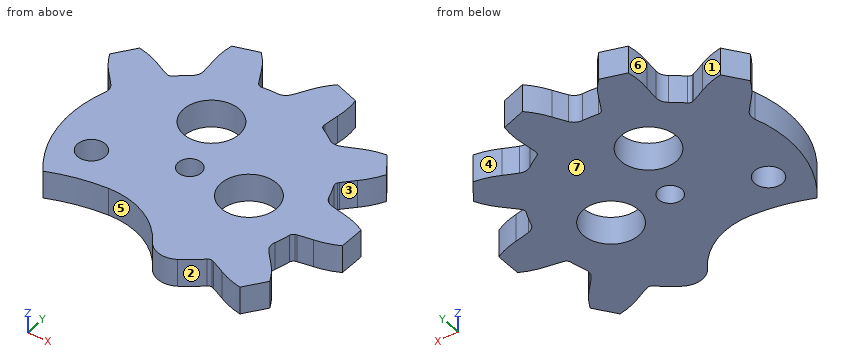
from build123d import *

# Parameters (mm, degrees)
ESQUISSE1_R        = 1.25
ESQUISSE1_R_2      = 3
ESQUISSE1_R_3      = 1.5
BOSS_EXTRU_1_DEPTH = 3


with BuildPart() as part:
    # Esquisse1 → Boss.-Extru.1 (new body)
    with BuildSketch(Plane.XY):
        with BuildLine():
            Line((1036.168665086, 2163.92668469), (1038.777951956, 2164.735581239))
            ThreePointArc((1038.777951956, 2164.735581239), (1039.645641159, 2163.718776789), (1040.340855862, 2162.577088409))
            ThreePointArc((1040.340855862, 2162.577088409), (1040.710583065, 2161.870292972), (1041.100970281, 2161.174695519))
            ThreePointArc((1041.100970281, 2161.174695519), (1041.148071574, 2161.099838925), (1041.200361208, 2161.028509858))
            ThreePointArc((1041.200361208, 2161.028509858), (1041.401673575, 2160.876243049), (1041.651712938, 2160.841715271))
            ThreePointArc((1041.651712938, 2160.841715271), (1042.472135802, 2160.912263521), (1043.295397124, 2160.929913601))
            ThreePointArc((1043.295397124, 2160.929913601), (1043.910230031, 2161.084508602), (1044.369546036, 2161.521484488))
            ThreePointArc((1044.369546036, 2161.521484488), (1044.778634779, 2162.206250429), (1045.167374464, 2162.902769957))
            ThreePointArc((1045.167374464, 2162.902769957), (1045.893264106, 2164.025204841), (1046.788181642, 2165.01812903))
            Line((1046.788181642, 2165.01812903), (1049.374596526, 2164.138839743))
            ThreePointArc((1049.374596526, 2164.138839743), (1049.478909177, 2162.806212746), (1049.370282093, 2161.473930495))
            ThreePointArc((1049.370282093, 2161.473930495), (1049.25395375, 2160.684800777), (1049.160921717, 2159.892586769))
            ThreePointArc((1049.160921717, 2159.892586769), (1049.155027862, 2159.804341066), (1049.155404891, 2159.715899564))
            ThreePointArc((1049.155404891, 2159.715899564), (1049.228769832, 2159.474384686), (1049.410761007, 2159.299481677))
            ThreePointArc((1049.410761007, 2159.299481677), (1050.115964268, 2158.874323951), (1050.792371125, 2158.404702301))
            ThreePointArc((1050.792371125, 2158.404702301), (1051.380650057, 2158.168382569), (1052.009092492, 2158.251924312))
            ThreePointArc((1052.009092492, 2158.251924312), (1052.742547559, 2158.565455267), (1053.466448477, 2158.900455947))
            ThreePointArc((1053.466448477, 2158.900455947), (1054.713456205, 2159.381857617), (1056.021085895, 2159.65913083))
            Line((1056.021085895, 2159.65913083), (1057.596706215, 2157.42751433))
            ThreePointArc((1057.596706215, 2157.42751433), (1056.897798427, 2156.288083004), (1056.026821411, 2155.274093419))
            ThreePointArc((1056.026821411, 2155.274093419), (1055.468870995, 2154.704050151), (1054.927954788, 2154.117818412))
            ThreePointArc((1054.927954788, 2154.117818412), (1054.871317037, 2154.04989046), (1054.819637448, 2153.97811817))
            ThreePointArc((1054.819637448, 2153.97811817), (1054.73703205, 2153.739605699), (1054.781460594, 2153.491134464))
            ThreePointArc((1054.781460594, 2153.491134464), (1055.102080574, 2152.732666561), (1055.373268538, 2151.955152691))
            ThreePointArc((1055.373268538, 2151.955152691), (1055.710290937, 2151.41818433), (1056.267816152, 2151.116381825))
            ThreePointArc((1056.267816152, 2151.116381825), (1057.045482637, 2150.938919624), (1057.828039241, 2150.784442585))
            ThreePointArc((1057.828039241, 2150.784442585), (1059.119850487, 2150.440931965), (1060.340722234, 2149.896645259))
            Line((1060.340722234, 2149.896645259), (1060.303714582, 2147.165103197))
            ThreePointArc((1060.303714582, 2147.165103197), (1059.068545375, 2146.654091582), (1057.767902043, 2146.34570422))
            ThreePointArc((1057.767902043, 2146.34570422), (1056.981447648, 2146.212484556), (1056.199258874, 2146.056155685))
            ThreePointArc((1056.199258874, 2146.056155685), (1056.113510922, 2146.034491652), (1056.029514563, 2146.006803149))
            ThreePointArc((1056.029514563, 2146.006803149), (1055.822491279, 2145.862396742), (1055.712386998, 2145.635264847))
            ThreePointArc((1055.712386998, 2145.635264847), (1055.525957764, 2144.833195728), (1055.288342248, 2144.044773508))
            ThreePointArc((1055.288342248, 2144.044773508), (1055.245377014, 2143.412260183), (1055.519029326, 2142.840391728))
            ThreePointArc((1055.519029326, 2142.840391728), (1056.043865064, 2142.239720901), (1056.58616733, 2141.65477112))
            ThreePointArc((1056.58616733, 2141.65477112), (1057.429354105, 2140.617557591), (1058.097136398, 2139.459609988))
            Line((1058.097136398, 2139.459609988), (1056.461636439, 2137.271498592))
            ThreePointArc((1056.461636439, 2137.271498592), (1055.161998468, 2137.584095755), (1053.928490366, 2138.099104107))
            ThreePointArc((1053.928490366, 2138.099104107), (1053.21393084, 2138.45359343), (1052.489239025, 2138.786879742))
            ThreePointArc((1052.489239025, 2138.786879742), (1052.407133676, 2138.819754553), (1052.3229043, 2138.846725905))
            ThreePointArc((1052.3229043, 2138.846725905), (1052.070538988, 2138.851583901), (1051.847957976, 2138.73254801))
            ThreePointArc((1051.847957976, 2138.73254801), (1050.855746376, 2137.899121153), (1049.782953643, 2137.172347506))
            ThreePointArc((1049.782953643, 2137.172347506), (1048.021944621, 2136.890714387), (1046.562157009, 2137.915160637))
            ThreePointArc((1046.562157009, 2137.915160637), (1043.357692527, 2140.785881782), (1039.138805682, 2141.628868317))
            ThreePointArc((1039.138805682, 2141.628868317), (1036.064607347, 2141.162614564), (1033.106023732, 2140.206125696))
            ThreePointArc((1033.106023732, 2140.206125696), (1030.545439739, 2145.948051891), (1031.027624755, 2152.216528933))
            ThreePointArc((1031.027624755, 2152.216528933), (1031.07058999, 2152.849042258), (1030.796937677, 2153.420910712))
            ThreePointArc((1030.796937677, 2153.420910712), (1030.27210194, 2154.02158154), (1029.729799674, 2154.606531321))
            ThreePointArc((1029.729799674, 2154.606531321), (1028.886612898, 2155.643744849), (1028.218830606, 2156.801692452))
            Line((1028.218830606, 2156.801692452), (1029.854330565, 2158.989803849))
            ThreePointArc((1029.854330565, 2158.989803849), (1031.153968536, 2158.677206686), (1032.387476638, 2158.162198333))
            ThreePointArc((1032.387476638, 2158.162198333), (1033.102036163, 2157.807709011), (1033.826727979, 2157.474422698))
            ThreePointArc((1033.826727979, 2157.474422698), (1033.908833328, 2157.441547887), (1033.993062704, 2157.414576536))
            ThreePointArc((1033.993062704, 2157.414576536), (1034.245428015, 2157.40971854), (1034.468009028, 2157.52875443))
            ThreePointArc((1034.468009028, 2157.52875443), (1035.090277846, 2158.068061624), (1035.74593579, 2158.566241703))
            ThreePointArc((1035.74593579, 2158.566241703), (1036.152477399, 2159.052701401), (1036.267223872, 2159.676201493))
            ThreePointArc((1036.267223872, 2159.676201493), (1036.195688295, 2160.470645106), (1036.1007814, 2161.262636695))
            ThreePointArc((1036.1007814, 2161.262636695), (1036.028287785, 2162.597372817), (1036.168665086, 2163.92668469))
        make_face()
        with Locations((1043.15798434, 2148.13065004)):
            Circle(ESQUISSE1_R, mode=Mode.SUBTRACT)
        with Locations((1040.931477639, 2154.395616576)):
            Circle(ESQUISSE1_R_2, mode=Mode.SUBTRACT)
        with Locations((1049.629972316, 2147.99435183)):
            Circle(ESQUISSE1_R_2, mode=Mode.SUBTRACT)
        with Locations((1034.806177599, 2145.042773361)):
            Circle(ESQUISSE1_R_3, mode=Mode.SUBTRACT)
    extrude(amount=BOSS_EXTRU_1_DEPTH)


solid = part.part
Source: CAD feature listing. Evaluate the final solid. Frame: model axes, mm. Face numbers are marked on the shaded views. A direction names the side the tool comes from. Round coordinates to 2 decimals unless told otherwise and drop trailing zeros. Write each loop counter-clockwise with the first axis right and the second up, starting at its lowest first coordinate (ties: lowest second). Pieces come first, ordered by that corner, then holes. Notation, with made-up numbers: (-34, -39) - (-19, -39) arc R18 cw to (-19, -30) - close; hole circle Ø3 at (-13, -2.5). An arc over 180 degrees is marked (long way). Use CSV: the item, a comma, the result in double quotes. Start each with the question number.
(1) Material intervals for probe 1 along Y at (x, z) = (1043, 1.5); probe 2 along Y at (x, z) = (1042.5, 0.9); probe 3 along X at (y, z) = (2159.75, 0.75), sorted ascending. Write a range as [from, to].
(2) Mould query, pull axis X, two halves, no side actions, for the marked faces 4, 5, 6 and 7. Classes: pulls with the +X half, pulls with the -X half, needs draft (parallel to the pull), parting line crosses it, or undercut.
(3) Cut plane A-A, the plane x = 1048. Return loops of the section in (y, z), and give its area (3 significant figures).
(4) Cut plane B-B, the plane x = 1057. Return loops of the section in (y, z).
(5) First-contact query: pin 1 Ø1 at (y, z) = (2150.5, 1.5) entering from -X; pin 2 Ø1 at (x, z) = (1042.5, 1) entering from +Y; pin 3 Ø1.5 at (y, z) = (2146, 0.5) entering from -X. Flat tips, straight axial feed; report the tip coordinate or a pass-through.
(6) Set-up query: the marked faces 1, 2 and 3. Return all of +Z, -Z, +X, -X, +Y, -Y with unobstructed straight access to the full face (end or side cutting, diameter ignored); none if empty.
(7) Cut plane C-C, the plane z = 2.5. Give the number of separate pieces and of enclosed holes in the cut face, and give its area (3 significant figures).
Geometry says:
1,probe 1,"[2140.95, 2146.89], [2149.37, 2152.22], [2156.57, 2160.93]"
1,probe 2,"[2141.16, 2147.07], [2149.19, 2151.84], [2156.95, 2160.91]"
1,probe 3,"[1036.26, 1049.15]"
2,face 4,"undercut"
2,face 5,"undercut"
2,face 6,"pulls with the -X half"
2,face 7,"needs draft"
3,outline,"(2136.9, 0) - (2145.48, 0) - (2145.48, 3) - (2136.9, 3) - close; (2150.51, 0) - (2164.61, 0) - (2164.61, 3) - (2150.51, 3) - close"
3,area,"68.0 mm²"
4,outline,"(2137.99, 0) - (2141.19, 0) - (2141.19, 3) - (2137.99, 3) - close; (2146.22, 0) - (2150.95, 0) - (2150.95, 3) - (2146.22, 3) - close; (2156.43, 0) - (2158.27, 0) - (2158.27, 3) - (2156.43, 3) - close"
5,pin 1,"x = 1030.5"
5,pin 2,"y = 2160.93"
5,pin 3,"x = 1030.43"
6,face 1,"+Z, -Z, +Y"
6,face 2,"+Z, -Z, -Y"
6,face 3,"+Z, -Z, +X"
7,separate pieces,"1"
7,enclosed holes,"4"
7,area,"499 mm²"
